from build123d import *

# Parameters (mm, degrees)
SKETCH_1_W          = 21.1
SKETCH_1_H          = 43.5
EXTRUDE_1_DEPTH     = 1.5
SKETCH_6_R          = 1.5
SKETCH_6_R_2        = 0.6
CUT_EXTRUDE_2_DEPTH = 1.5
SKETCH_7_R          = 4
EXTRUDE_9_DEPTH     = 11
EXTRUDE_10_DEPTH    = 8
SKETCH_7_4_W        = 8.5
SKETCH_7_4_H        = 9.5
EXTRUDE_11_DEPTH    = 4.5
FILLET_1_R          = 0.5
SKETCH_4_3_W        = 4.5
SKETCH_4_3_H        = 9.5
EXTRUDE_7_DEPTH     = 10
EXTRUDE_START       = 10
SKETCH_4_3_3_R      = 1.15
EXTRUDE_8_DEPTH     = 1.6
SKETCH_5_W          = 0.6
SKETCH_5_H          = 3
CUT_EXTRUDE_1_DEPTH = 0.5


with BuildPart() as part:
    # Sketch 1 → Extrude 1 (new body)
    with BuildSketch(Plane.XY):
        Rectangle(SKETCH_1_W, SKETCH_1_H)
    extrude(amount=EXTRUDE_1_DEPTH)

    # Sketch 6 → Cut-Extrude 2 (cut)
    with BuildSketch(Plane.XY.offset(1.5)):
        with Locations((8.01, 15.15)):
            Circle(SKETCH_6_R)
        with Locations((-8.01, -15.15)):
            Circle(SKETCH_6_R)
        with Locations((9.05, 20.25)):
            Circle(SKETCH_6_R_2)
        with Locations(Location((-9.05, 20.25, 0), (0, 0, 180))):
            Circle(SKETCH_6_R_2)
        with Locations(Location((9.05, -20.25, 0), (0, 0, 180))):
            Circle(SKETCH_6_R_2)
        with Locations((-9.05, -20.25)):
            Circle(SKETCH_6_R_2)
    extrude(amount=-CUT_EXTRUDE_2_DEPTH, mode=Mode.SUBTRACT)

    # Sketch 7 → Extrude 9 (add)
    with BuildSketch(Plane.XY.offset(1.5)):
        with Locations(Location((0, 17.35, 0), (0, 0, 180))):
            Circle(SKETCH_7_R)
        with Locations((0, -17.35)):
            Circle(SKETCH_7_R)
    extrude(amount=EXTRUDE_9_DEPTH)

    # Sketch 7_3 → Extrude 10 (add)
    with BuildSketch(Plane.XY.offset(1.5)):
        with BuildLine():
            ThreePointArc((8.55, 11.65), (9.257106781, 11.357106781), (9.55, 10.65))
            Line((9.55, 10.65), (9.55, 0.45))
            ThreePointArc((9.55, 0.45), (9.257106781, -0.257106781), (8.55, -0.55))
            Line((8.55, -0.55), (-1.65, -0.55))
            ThreePointArc((-1.65, -0.55), (-2.357106781, -0.257106781), (-2.65, 0.45))
            Line((-2.65, 0.45), (-2.65, 10.65))
            ThreePointArc((-2.65, 10.65), (-2.357106781, 11.357106781), (-1.65, 11.65))
            Line((-1.65, 11.65), (8.55, 11.65))
        make_face()
    extrude(amount=EXTRUDE_10_DEPTH)

    # Sketch 7_4 → Extrude 11 (add)
    with BuildSketch(Plane.XY.offset(1.5)):
        with Locations((-4.3, -7)):
            Rectangle(SKETCH_7_4_W, SKETCH_7_4_H)
    extrude(amount=EXTRUDE_11_DEPTH)

    # Fillet 1
    fillet_1_edges = [part.edges().sort_by_distance(p)[0] for p in [
        (4, 17.35, 12.5),
        (-4, -17.35, 12.5),
    ]]
    fillet(fillet_1_edges, radius=FILLET_1_R)



with BuildPart() as body_2:
    # Sketch 4_3 → Extrude 7 (new body)
    with BuildSketch(Plane(origin=(5.475455411, 30.634305543, 1.5), x_dir=(1, 0, 0), z_dir=(0, 0, 1))):
        with Locations((-12.775455411, -23.334305543)):
            Rectangle(SKETCH_4_3_W, SKETCH_4_3_H)
    extrude(amount=EXTRUDE_7_DEPTH)


with BuildPart() as part_1:
    add(part.part)

    add(body_2.part)  # Extrude 8 merges body 2
    # Sketch 4_3_3 → Extrude 8 (add)
    with BuildSketch(Plane(origin=(5.475455411, 30.634305543, 1.5), x_dir=(1, 0, 0), z_dir=(0, 0, 1)).offset(EXTRUDE_START)):
        with Locations(Location((-13.875455411, -26.934305543, 0), (0, 0, 180))):
            Circle(SKETCH_4_3_3_R)
    extrude(amount=EXTRUDE_8_DEPTH)

    # Sketch 5 → Cut-Extrude 1 (cut)
    with BuildSketch(Plane(origin=(6.95, -7.75, 13.1), x_dir=(1, 0, 0), z_dir=(0, 0, 1))):
        with Locations((-15.35, 11.45)):
            Rectangle(SKETCH_5_W, SKETCH_5_H)
    extrude(amount=-CUT_EXTRUDE_1_DEPTH, mode=Mode.SUBTRACT)


solid = part_1.part
Design review of the part built by this model. Coordinates are the model's own, in mm. A direction names the side the tool comes from. Round coordinates to 2 decimals unless told otherwise and drop trailing zeros. Order: outer loops, then holes, each group sorted by start corner. A loop starts at its lowest first (then second) coordinate and runs counter-clockwise, first axis right, second up.
1) Draft analysis for pull direction X (two halves, no side actions). For faces 5 (the cylindrical face through (-0.867, -21.255, 6.676)), 6 (the flat face through (0, -21.75, 1)), 7 (the cylindrical face through (-8.972, 19.655, 0.76)), 8 (the flat face through (-0.05, -7, 4)), state which applies: released by +X, released by -X, zero draft, split by the parting line, or undercut.
The answers:
face 5: split by the parting line
face 6: zero draft
face 7: undercut
face 8: released by +X
2) Machinability: for faces 1 (the flat face through (9.55, 6, 5)), 2 (the flat face through (4, -0.55, 5)), 3 (the flat face through (-7, 2.55, 6)), 4 (the cylindrical face through (-2.365, 11.349, 5.444)), which of the approach directions +Z, -Z, +X, -X, +Y, -Y give a long, thin tool a straight path to every point of the face, cutting with its end or side? Answer none if there is none.
The answers:
face 1: +Z, +X, +Y, -Y
face 2: +Z, +X, -X
face 3: +Z, -X
face 4: +Z
3) Consider section D-D (x = 9.05). State the section outline as (y, z) points.
The answers:
outline: (-21.75, 0) - (-20.85, 0) - (-20.85, 1.5) - (-21.75, 1.5) - close; (-19.65, 0) - (14.07, 0) - (14.07, 1.5) - (11.52, 1.5) - (11.52, 9.5) - (-0.42, 9.5) - (-0.42, 1.5) - (-19.65, 1.5) - close; (16.23, 0) - (19.65, 0) - (19.65, 1.5) - (16.23, 1.5) - close; (20.85, 0) - (21.75, 0) - (21.75, 1.5) - (20.85, 1.5) - close
4) For L1, parallel to Y at x = -1, z = 8; L2, parallel to Y at x = -8.01, z = 1; L3, parallel to Z at x = -7, y = 20, list the stretches that pass through material, from the lowest coordinate up.
The answers:
L1: y = -21.22 to -13.48, -0.55 to 11.65, 13.48 to 21.22
L2: y = -21.75 to -16.65, -13.65 to 21.75
L3: z = 0 to 1.5
5) Consider section C-C (z = 3.5). State the section outline as (x, y) points.
The answers:
outline: (-9.55, 2.55) - (-5.05, 2.55) - (-5.05, 12.05) - (-9.55, 12.05) - close; (-8.55, -11.75) - (-0.05, -11.75) - (-0.05, -2.25) - (-8.55, -2.25) - close; circle Ø8 at (0, -17.35); circle Ø8 at (0, 17.35); (-2.65, 0.45) arc R1 ccw to (-1.65, -0.55) - (8.55, -0.55) arc R1 ccw to (9.55, 0.45) - (9.55, 10.65) arc R1 ccw to (8.55, 11.65) - (-1.65, 11.65) arc R1 ccw to (-2.65, 10.65) - close
6) Consider section A-A (z = 8.75). State the section outline as (x, y) points.
The answers:
outline: (-9.55, 2.55) - (-5.05, 2.55) - (-5.05, 12.05) - (-9.55, 12.05) - close; circle Ø8 at (0, -17.35); circle Ø8 at (0, 17.35); (-2.65, 0.45) arc R1 ccw to (-1.65, -0.55) - (8.55, -0.55) arc R1 ccw to (9.55, 0.45) - (9.55, 10.65) arc R1 ccw to (8.55, 11.65) - (-1.65, 11.65) arc R1 ccw to (-2.65, 10.65) - close
7) Clearance check with flat-ended pins moving along their axes: pin 1 Ø2 at (x, z) = (7.5, 5.5) entering from -Y; pin 2 Ø1.3 at (x, z) = (-3.5, 3.5) entering from -Y; pin 3 Ø1.3 at (x, z) = (-7, 5) entering from -Y; pin 4 Ø5 at (y, z) = (-9, 2.5) entering from -X. State where each tip first meets the part, or that it passes through.
The answers:
pin 1: stops at y = -0.55
pin 2: stops at y = -20.16
pin 3: stops at y = -11.75
pin 4: stops at x = -10.55
8) Consider section B-B (y = -8). State the section outline as (x, z) points, plus the area to 3 significant figures.
The answers:
outline: (-10.55, 0) - (10.55, 0) - (10.55, 1.5) - (-0.05, 1.5) - (-0.05, 6) - (-8.55, 6) - (-8.55, 1.5) - (-10.55, 1.5) - close
area: 69.9 mm2
